Part model, mm, in its own coordinate system. Face numbers are marked on the shaded views. A direction names the side the tool comes from. Round coordinates to 2 decimals unless told otherwise and drop trailing zeros. Write each loop counter-clockwise with the first axis right and the second up, starting at its lowest first coordinate (ties: lowest second). Pieces come first, ordered by that corner, then holes. Notation, with made-up numbers: M 57,-29 L 83,-29 A7 ccw 83,-22 Z; hole C 17,48.5 d5. An arc over 180 degrees is marked long. Use a Markdown table: item, result. Add a question column.
1) Which spindle directions (+Z, -Z, +X, -X, +Y, -Y) get a long thin tool onto all of the face, cutting with end or side? Do the marked faces 4, 5, 6 and 7. Say none if no direction does.
2) Drop flat-ended pins along their axis: P1, Ø4, axis at x = 18.5, y = 168.5, coming from the -Z side; P2, Ø1.5, axis at y = 49, z = -30, coming from the -X side; P3, Ø1, axis at x = 43.5, y = 92.5, coming from the +Z side. Give the stop position or say it passes through.
3) Slice it at C-C on z = 12. Write the cut outline in (x, y).
4) Slice it at D-D on x = 50. Write the cut outline in (y, z).
5) Slice it at A-A on x = 3. Write the cut outline in (y, z), plus the area to 3 significant figures.
6) Slice it at B-B on y = 64. Write the cut outline in (x, z), plus the area to 3 significant figures.
7) Wall check: probe 1 along X at (y, z) = (50, 32); probe 2 along Y at (x, z) = (-39.5, -2); probe 3 along Y at (x, z) = (-54.5, 48). Give the ranges that are in metal, low to high.
8) Two-plate mould, pull along X, no slides. Class the marked faces 1, 2 and 3: released by +X, released by -X, zero draft, split by the parting line, or undercut.
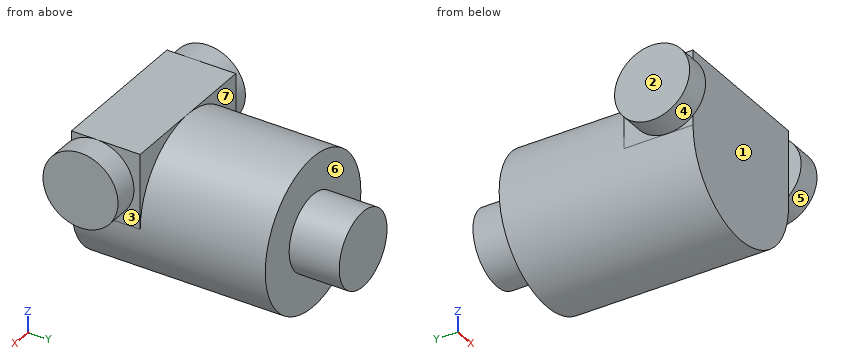
```python
from build123d import *

# Parameters (mm, degrees)
ESQUISSE2_W        = 120
ESQUISSE2_H        = 60
BOSS_EXTRU_1_DEPTH = 55
ESQUISSE3_R        = 30
BOSS_EXTRU_2_DEPTH = 20


with BuildPart() as part:
    # Esquisse1 → Révolution1 (revolve)
    with BuildSketch(Plane.XY):
        Polygon((0, 0), (-60, 0), (-60, 155), (-30, 155), (-30, 195), (0, 195), align=None)
    revolve(axis=Axis((0, 195, 0), (0, -1, 0)))

    # Esquisse2 → Boss.-Extru.1 (add)
    with BuildSketch(Plane.XZ):
        with Locations((0, 30)):
            Rectangle(ESQUISSE2_W, ESQUISSE2_H)
    extrude(amount=-BOSS_EXTRU_1_DEPTH)

    # Esquisse3 → Boss.-Extru.2 (add)
    with BuildSketch(Plane.ZY.offset(60)):
        with Locations((30, 20)):
            Circle(ESQUISSE3_R)
    boss_extru_2 = extrude(amount=BOSS_EXTRU_2_DEPTH)

    # Symétrie1: Boss.-Extru.2 across plane
    add(boss_extru_2.mirror(Plane(origin=(0, 0, 0), x_dir=(0, 0, 1), z_dir=(1, 0, 0))))


solid = part.part
```
Entries:
| question | item | result |
|---|---|---|
| 1 | face 4 | -X |
| 1 | face 5 | +X |
| 1 | face 6 | +Y |
| 1 | face 7 | +Z, -X, +Y |
| 2 | P1 | stops at z = -25.05 |
| 2 | P2 | stops at x = -52.39 |
| 2 | P3 | stops at z = 41.84 |
| 3 | outline | M -80,-4 L -60,-4 L -60,0 L 60,0 L 60,-4 L 80,-4 L 80,44 L 60,44 L 60,55 L 58.79,55 L 58.79,155 L 27.5,155 L 27.5,195 L -27.5,195 L -27.5,155 L -58.79,155 L -58.79,55 L -60,55 L -60,44 L -80,44 Z |
| 4 | outline | M 0,-33.17 L 155,-33.17 L 155,33.17 L 55,33.17 L 55,60 L 0,60 Z |
| 5 | outline | M 0,-59.92 L 155,-59.92 L 155,-29.85 L 195,-29.85 L 195,29.85 L 155,29.85 L 155,59.92 L 55,59.92 L 55,60 L 0,60 Z |
| 5 | area | 21,000 mm^2 |
| 6 | outline | C 0,0 d120 |
| 6 | area | 11,300 mm^2 |
| 7 | probe 1 | x = -60 to 60 |
| 7 | probe 2 | y = 0 to 155 |
| 7 | probe 3 | y = 0 to 55 |
| 8 | face 1 | undercut |
| 8 | face 2 | released by -X |
| 8 | face 3 | released by +X |
